Geometry check sheet. Reference: the model listing, model coordinates, mm. A direction names the side the tool comes from. Round coordinates to 2 decimals unless told otherwise and drop trailing zeros. Order: outer loops, then holes, each group sorted by start corner. A loop starts at its lowest first (then second) coordinate and runs counter-clockwise, first axis right, second up. Notation, with made-up numbers: (4.5, -27) - (63.5, -27) arc R21 ccw to (63.5, 7) - close; hole circle Ø11 at (26, 73.5). An arc over 180 degrees is marked (long way). Use a Markdown table: item, result. Add a question column.
(1) Section check C-C on x = -6. Record the boundary of the cut face in (y, z).
(2) Mould release check, pull along X, two halves, no side actions. Record for faces 1 (the face through (-1, -58, 4)), 2 (the face through (-47.286, -26.869, 9.433)), 3 (the face through (-41, -44, 2)): released by +X, released by -X, zero draft, split by the parting line, or undercut.
(3) Section check A-A on x = 37.62. Record the boundary of the cut face in (y, z).
(4) Gauge pin test, flat ends, axial feed: P1, Ø1.5, axis at x = -46.5, z = 1, coming from the +Y side; P2, Ø3.5, axis at x = -37.62, y = -25, coming from the +Z side; P3, Ø1.3, axis at x = -46.5, y = 36, coming from the +Z side. Record the tip position at first contact, or that the pin passes through.
(5) Section check D-D on y = -4. Record the boundary of the cut face in (x, z).
(6) Section check B-B on y = -30.88. Record the boundary of the cut face in (x, z).
(7) Access from +Z, -Z, +X, -X, +Y, -Y to the whole of each face (thin tool, end or side, straight path). Record for faces 4 (the face through (-20, 37, 7)), 5 (the face through (-5, 35, 2.5)), 6 (the face through (6, 39.2, 9)), 7 (the face through (18, 22, 3.25)), 8 (the face through (39, -4, 3)).
(8) Thickness scan on line 1 along Y through (x, z) = (20.38, 4); line 2 along Y through (x, z) = (45.5, 12.1); line 3 along Y through (x, z) = (18.25, 1.2). Record the ranges inside material, lowest first. Write a range as [from, to].
```python
from build123d import *

# Parameters (mm, degrees)
SKETCH1_W                                       = 98
SKETCH1_H                                       = 80
BOSS_EXTRUDE1_DEPTH                             = 5
SKETCH2_W                                       = 7
SKETCH2_H                                       = 80
BOSS_EXTRUDE2_DEPTH                             = 8.5
SKETCH3_W                                       = 7
SKETCH3_H                                       = 80
BOSS_EXTRUDE3_DEPTH                             = 8.5
SKETCH8_W                                       = 84
SKETCH8_H                                       = 8.5
BOSS_EXTRUDE5_DEPTH                             = 5
SKETCH13_R                                      = 2.25
CUT_EXTRUDE7_DEPTH                              = 3.25
SKETCH15_R                                      = 1.5
CUT_EXTRUDE9_DEPTH                              = 3.25
SKETCH14_W                                      = 16
SKETCH14_H                                      = 16
CUT_EXTRUDE13_DEPTH                             = 3
SKETCH18_W                                      = 16
SKETCH18_H                                      = 12
CUT_EXTRUDE14_DEPTH                             = 64.822018144
SKETCH19_W                                      = 16
SKETCH19_H                                      = 5.672791846
CUT_EXTRUDE15_DEPTH                             = 3
SKETCH20_R                                      = 2.25
CUT_EXTRUDE20_DEPTH                             = 3.25
BOSS_EXTRUDE7_DEPTH                             = 10
BOSS_EXTRUDE9_DEPTH                             = 8
CSK_FOR_M3_FLAT_HEAD_MACHINE_SCREW1_D           = 3.4
CSK_FOR_M3_FLAT_HEAD_MACHINE_SCREW1_CSINK_D     = 6.3
CSK_FOR_M3_FLAT_HEAD_MACHINE_SCREW1_CSINK_ANGLE = 90
SKETCH51_R                                      = 17.5
CUT_EXTRUDE23_DEPTH                             = 8
CUT_EXTRUDE24_START                             = -8
SKETCH52_R                                      = 17.5
CUT_EXTRUDE24_DEPTH                             = 8
SKETCH42_R                                      = 2.25
CUT_EXTRUDE25_DEPTH                             = 4.25
SKETCH53_R                                      = 2.25
CUT_EXTRUDE26_DEPTH                             = 8.25
SKETCH54_R                                      = 2.25
CUT_EXTRUDE27_DEPTH                             = 13.25
CUT_EXTRUDE28_DEPTH                             = 5
CUT_EXTRUDE29_START                             = -13.25
SKETCH56_R                                      = 2.25
CUT_EXTRUDE29_DEPTH                             = 13.25
CUT_EXTRUDE30_START                             = -5
CUT_EXTRUDE30_DEPTH                             = 5
SKETCH65_W                                      = 20.4
SKETCH65_H                                      = 14
CUT_EXTRUDE31_DEPTH                             = 77.401897882
SKETCH69_W                                      = 6
SKETCH69_H                                      = 6
CUT_EXTRUDE33_DEPTH                             = 13.5
SKETCH75_W                                      = 28.5
SKETCH75_H                                      = 7
CUT_EXTRUDE39_DEPTH                             = 11
SKETCH77_R                                      = 2.5
BOSS_EXTRUDE11_DEPTH                            = 2.5
SKETCH79_R                                      = 1.5
CUT_EXTRUDE41_DEPTH                             = 3.2
SKETCH80_W                                      = 5
SKETCH80_H                                      = 12
CUT_EXTRUDE42_DEPTH                             = 77.401897882
SKETCH82_W                                      = 0.8
SKETCH82_H                                      = 7
SKETCH82_W_2                                    = 0.2
CUT_EXTRUDE43_DEPTH                             = 11


with BuildPart() as part:
    # Sketch1 → Boss-Extrude1 (new body)
    with BuildSketch(Plane.XY):
        Rectangle(SKETCH1_W, SKETCH1_H)
    extrude(amount=BOSS_EXTRUDE1_DEPTH)

    # Sketch2 → Boss-Extrude2 (add)
    with BuildSketch(Plane.XY.offset(5)):
        with Locations((-45.5, 0)):
            Rectangle(SKETCH2_W, SKETCH2_H)
    extrude(amount=BOSS_EXTRUDE2_DEPTH)

    # Sketch3 → Boss-Extrude3 (add)
    with BuildSketch(Plane.XY.offset(5)):
        with Locations((45.5, 0)):
            Rectangle(SKETCH3_W, SKETCH3_H)
    extrude(amount=BOSS_EXTRUDE3_DEPTH)

    # Sketch8 → Boss-Extrude5 (add)
    with BuildSketch(Plane(origin=(0, 40, 0), x_dir=(1, 0, 0), z_dir=(0, 1, 0))):
        with Locations((0, -9.25)):
            Rectangle(SKETCH8_W, SKETCH8_H)
    extrude(amount=-BOSS_EXTRUDE5_DEPTH)

    # Sketch13 → Cut-Extrude7 (cut)
    with BuildSketch(Plane.XY.offset(5)):
        with Locations((0, -10)):
            Circle(SKETCH13_R)
    extrude(amount=-CUT_EXTRUDE7_DEPTH, mode=Mode.SUBTRACT)

    # Sketch15 → Cut-Extrude9 (cut)
    with BuildSketch(Plane.XY.offset(5)):
        with Locations((-37.62, 17)):
            Circle(SKETCH15_R)
        with Locations((-20.38, 17)):
            Circle(SKETCH15_R)
        with Locations((-37.62, -25)):
            Circle(SKETCH15_R)
        with Locations((-20.38, -25)):
            Circle(SKETCH15_R)
        with Locations((20.38, -25)):
            Circle(SKETCH15_R)
        with Locations((37.62, -25)):
            Circle(SKETCH15_R)
        with Locations((37.62, 17)):
            Circle(SKETCH15_R)
        with Locations((20.38, 17)):
            Circle(SKETCH15_R)
    extrude(amount=-CUT_EXTRUDE9_DEPTH, mode=Mode.SUBTRACT)

    # Sketch14 → Cut-Extrude13 (cut)
    with BuildSketch(Plane.XY.offset(5)):
        with Locations((0, 6.327208154)):
            Rectangle(SKETCH14_W, SKETCH14_H)
    extrude(amount=-CUT_EXTRUDE13_DEPTH, mode=Mode.SUBTRACT)

    # Sketch18 → Cut-Extrude14 (cut, through all)
    with BuildSketch(Plane.XY.offset(5)):
        with Locations((0, 26)):
            Rectangle(SKETCH18_W, SKETCH18_H)
    extrude(amount=-CUT_EXTRUDE14_DEPTH, mode=Mode.SUBTRACT)

    # Sketch19 → Cut-Extrude15 (cut)
    with BuildSketch(Plane.XY.offset(5)):
        with Locations((0, 17.163604077)):
            Rectangle(SKETCH19_W, SKETCH19_H)
    extrude(amount=-CUT_EXTRUDE15_DEPTH, mode=Mode.SUBTRACT)

    # Sketch20 → Cut-Extrude20 (cut)
    with BuildSketch(Plane(origin=(0, 0, 0), x_dir=(-1, 0, 0), z_dir=(0, 0, -1))):
        with Locations((18.25, 21.5)):
            Circle(SKETCH20_R)
        with Locations((-18.25, 21.5)):
            Circle(SKETCH20_R)
        with Locations((18.25, -15)):
            Circle(SKETCH20_R)
        with Locations((-18.25, -15)):
            Circle(SKETCH20_R)
    extrude(amount=-CUT_EXTRUDE20_DEPTH, mode=Mode.SUBTRACT)

    # Sketch26 → Boss-Extrude7 (add)
    with BuildSketch(Plane(origin=(0, -40, 0), x_dir=(-1, 0, 0), z_dir=(0, -1, 0))):
        Polygon((49, -13.5), (42, -13.5), (42, -5), (-42, -5), (-42, -13.5), (-49, -13.5), (-49, 0), (49, 0), align=None)
    extrude(amount=BOSS_EXTRUDE7_DEPTH)

    # Sketch47 → Boss-Extrude9 (add)
    with BuildSketch(Plane(origin=(0, -50, 0), x_dir=(-1, 0, 0), z_dir=(0, -1, 0))):
        Polygon((49, -13.5), (42, -13.5), (42, -5), (-42, -5), (-42, -13.5), (-49, -13.5), (-49, 0), (49, 0), align=None)
    extrude(amount=BOSS_EXTRUDE9_DEPTH)

    # CSK for M3 Flat Head Machine Screw1 (through all)
    with Locations(Plane.XY.offset(5)):
        with Locations((28, -30.88), (0, -30.88), (-28, -30.88)):
            CounterSinkHole(CSK_FOR_M3_FLAT_HEAD_MACHINE_SCREW1_D / 2, CSK_FOR_M3_FLAT_HEAD_MACHINE_SCREW1_CSINK_D / 2, counter_sink_angle=CSK_FOR_M3_FLAT_HEAD_MACHINE_SCREW1_CSINK_ANGLE)

    # Sketch51 → Cut-Extrude23 (cut)
    with BuildSketch(Plane.ZY.offset(49)):
        with Locations((-13, -44)):
            Circle(SKETCH51_R)
    extrude(amount=-CUT_EXTRUDE23_DEPTH, mode=Mode.SUBTRACT)

    # Sketch52 → Cut-Extrude24 (cut)
    with BuildSketch(Plane(origin=(49, 0, 0), x_dir=(0, 0, -1), z_dir=(1, 0, 0)).offset(CUT_EXTRUDE24_START)):
        with Locations((13, -44)):
            Circle(SKETCH52_R)
    extrude(amount=CUT_EXTRUDE24_DEPTH, mode=Mode.SUBTRACT)

    # Sketch42 → Cut-Extrude25 (cut)
    with BuildSketch(Plane.XY.offset(13.5)):
        with Locations((-45.5, 36.5)):
            Circle(SKETCH42_R)
        with Locations((45.5, 36.5)):
            Circle(SKETCH42_R)
    extrude(amount=-CUT_EXTRUDE25_DEPTH, mode=Mode.SUBTRACT)

    # Sketch53 → Cut-Extrude26 (cut)
    with BuildSketch(Plane.XY.offset(13.5)):
        with Locations((-45.5, -25.5)):
            Circle(SKETCH53_R)
        with Locations((45.5, -25.5)):
            Circle(SKETCH53_R)
    extrude(amount=-CUT_EXTRUDE26_DEPTH, mode=Mode.SUBTRACT)

    # Sketch54 → Cut-Extrude27 (cut)
    with BuildSketch(Plane.ZY.offset(49)):
        with Locations((3, 37)):
            Circle(SKETCH54_R)
    extrude(amount=-CUT_EXTRUDE27_DEPTH, mode=Mode.SUBTRACT)

    # Sketch55 → Cut-Extrude28 (cut)
    with BuildSketch(Plane.ZY.offset(49)):
        with BuildLine():
            Line((5.5, 37), (5.5, 40))
            Line((5.5, 40), (0, 40))
            Line((0, 40), (0, 34.5))
            Line((0, 34.5), (3, 34.5))
            ThreePointArc((3, 34.5), (4.767766953, 35.232233047), (5.5, 37))
        make_face()
    extrude(amount=-CUT_EXTRUDE28_DEPTH, mode=Mode.SUBTRACT)

    # Sketch56 → Cut-Extrude29 (cut)
    with BuildSketch(Plane(origin=(49, 0, 0), x_dir=(0, 0, -1), z_dir=(1, 0, 0)).offset(CUT_EXTRUDE29_START)):
        with Locations(Location((-3, 37, 0), (0, 0, 180))):
            Circle(SKETCH56_R)
    extrude(amount=CUT_EXTRUDE29_DEPTH, mode=Mode.SUBTRACT)

    # Sketch57 → Cut-Extrude30 (cut)
    with BuildSketch(Plane(origin=(49, 0, 0), x_dir=(0, 0, -1), z_dir=(1, 0, 0)).offset(CUT_EXTRUDE30_START)):
        with BuildLine():
            Line((-5.5, 37), (-5.5, 40))
            Line((-5.5, 40), (0, 40))
            Line((0, 40), (0, 34.5))
            Line((0, 34.5), (-3, 34.5))
            ThreePointArc((-3, 34.5), (-4.767766953, 35.232233047), (-5.5, 37))
        make_face()
    extrude(amount=CUT_EXTRUDE30_DEPTH, mode=Mode.SUBTRACT)

    # Sketch65 → Cut-Extrude31 (cut, through all)
    with BuildSketch(Plane.XY.offset(5)):
        with Locations((-29, -4)):
            Rectangle(SKETCH65_W, SKETCH65_H)
        with Locations((28.8, -4)):
            Rectangle(SKETCH65_W, SKETCH65_H)
    extrude(amount=-CUT_EXTRUDE31_DEPTH, mode=Mode.SUBTRACT)

    # Sketch69 → Cut-Extrude33 (cut)
    with BuildSketch(Plane.XZ.offset(-35)):
        with Locations((0, 9.25)):
            Rectangle(SKETCH69_W, SKETCH69_H)
    extrude(amount=-CUT_EXTRUDE33_DEPTH, mode=Mode.SUBTRACT)

    # Sketch75 → Cut-Extrude39 (cut)
    with BuildSketch(Plane.XY.offset(13.5)):
        with Locations((-4.95, 35)):
            Rectangle(SKETCH75_W, SKETCH75_H)
    extrude(amount=-CUT_EXTRUDE39_DEPTH, mode=Mode.SUBTRACT)

    # Sketch77 → Boss-Extrude11 (add)
    with BuildSketch(Plane.XZ.offset(-38.5)):
        with Locations(Location((6.3, 9.05, 0), (0, 0, 90))):
            Circle(SKETCH77_R)
        with Locations(Location((-16.2, 9.05, 0), (0, 0, 90))):
            Circle(SKETCH77_R)
    extrude(amount=BOSS_EXTRUDE11_DEPTH)

    # Sketch79 → Cut-Extrude41 (cut)
    with BuildSketch(Plane.XZ.offset(-36)):
        with Locations(Location((6.3, 9.05, 0), (0, 0, 270))):
            Circle(SKETCH79_R)
        with Locations(Location((-16.2, 9.05, 0), (0, 0, 270))):
            Circle(SKETCH79_R)
    extrude(amount=-CUT_EXTRUDE41_DEPTH, mode=Mode.SUBTRACT)

    # Sketch80 → Cut-Extrude42 (cut, through all)
    with BuildSketch(Plane.XY.offset(5)):
        with Locations((-10.5, 26)):
            Rectangle(SKETCH80_W, SKETCH80_H)
    extrude(amount=-CUT_EXTRUDE42_DEPTH, mode=Mode.SUBTRACT)

    # Sketch82 → Cut-Extrude43 (cut)
    with BuildSketch(Plane.XY.offset(13.5)):
        with Locations((-19.6, 35)):
            Rectangle(SKETCH82_W, SKETCH82_H)
        with Locations((9.4, 35)):
            Rectangle(SKETCH82_W_2, SKETCH82_H)
    extrude(amount=-CUT_EXTRUDE43_DEPTH, mode=Mode.SUBTRACT)


solid = part.part
```
Check sheet entries:
| question | item | result |
|---|---|---|
| 1 | outline | (-58, 0) - (20, 0) - (20, 2) - (-1.67, 2) - (-1.67, 5) - (-58, 5) - close; (32, 0) - (40, 0) - (40, 13.5) - (38.5, 13.5) - (38.5, 2.5) - (32, 2.5) - close |
| 2 | face 1 | zero draft |
| 2 | face 2 | undercut |
| 2 | face 3 | released by -X |
| 3 | outline | (-58, 0) - (-11, 0) - (-11, 5) - (-23.5, 5) - (-23.5, 1.75) - (-26.5, 1.75) - (-26.5, 5) - (-58, 5) - close; (3, 0) - (40, 0) - (40, 13.5) - (35, 13.5) - (35, 5) - (18.5, 5) - (18.5, 1.75) - (15.5, 1.75) - (15.5, 5) - (3, 5) - close; hole circle Ø4.5 at (37, 3) |
| 4 | P1 | stops at y = 34.5 |
| 4 | P2 | stops at z = 5 |
| 4 | P3 | stops at z = 9.25 |
| 5 | outline | (-49, 0) - (-39.2, 0) - (-39.2, 5) - (-42, 5) - (-42, 13.5) - (-49, 13.5) - close; (-18.8, 0) - (18.6, 0) - (18.6, 5) - (-18.8, 5) - close; (39, 0) - (49, 0) - (49, 13.5) - (42, 13.5) - (42, 5) - (39, 5) - close |
| 6 | outline | (-49, 0) - (-29.7, 0) - (-29.7, 3.55) - (-31.15, 5) - (-42, 5) - (-42, 13.5) - (-49, 13.5) - close; (-26.3, 0) - (-1.7, 0) - (-1.7, 3.55) - (-3.15, 5) - (-24.85, 5) - (-26.3, 3.55) - close; (1.7, 0) - (26.3, 0) - (26.3, 3.55) - (24.85, 5) - (3.15, 5) - (1.7, 3.55) - close; (29.7, 0) - (49, 0) - (49, 13.5) - (42, 13.5) - (42, 5) - (31.15, 5) - (29.7, 3.55) - close |
| 7 | face 4 | +Z |
| 7 | face 5 | none |
| 7 | face 6 | -Y |
| 7 | face 7 | -Z |
| 7 | face 8 | +Z, -Z |
| 8 | line 1 | y = [-58, -26.5], [-23.5, -11], [3, 15.5], [18.5, 40] |
| 8 | line 2 | y = [-58, -27.75], [-23.25, 34.25], [38.75, 40] |
| 8 | line 3 | y = [-58, -17.25], [-12.75, 19.25], [23.75, 40] |
